Verification items for this drawing (mm, ordinates from the low corner). Give positions to 0.01 mm unless a question says otherwise; leave off trailing zeros. Loops run counter-clockwise (first coordinate to the right, second up) from the corner with the lowest first, then second, coordinate; pieces in that order, holes last. Notation, with made-up numbers: (44, -32) -> (94, -32) arc R16 cw to (94, -2) -> close; hole circle Ø2 at (83.5, 33). An arc over 180 degrees is marked (long way). Answer as a JSON object with one key per item and string values.
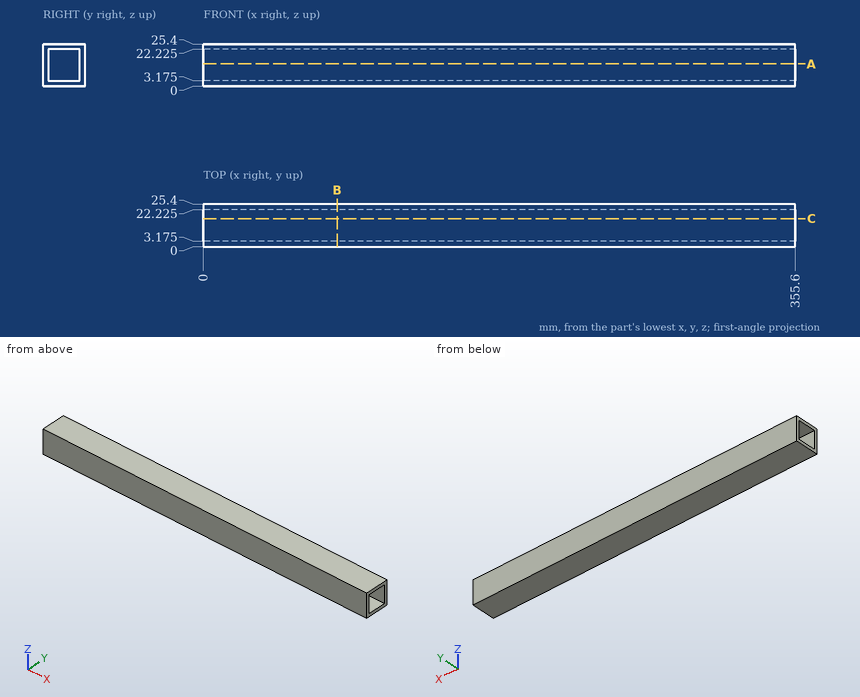
1) Depth check by flat-ended pin: P1, Ø10, axis at y = 18.5, z = 5, coming from the -X side. Enter the tip coordinate at first touch or a pass-through.
Geometry check:
{"P1": "stops at x = 0"}
2) Section check B-B on x = 80.5. Record the cut outline in (y, z) (3 decimals).
Geometry check:
{"outline": "(0, 0) -> (25.4, 0) -> (25.4, 25.4) -> (0, 25.4) -> close; hole (3.175, 3.175) -> (22.225, 3.175) -> (22.225, 22.225) -> (3.175, 22.225) -> close"}
3) Material ranges on line 1 along Y through (x, z) = (73, 21.75) (3 decimals), recorded low to high. Write a range as from..to.
Geometry check:
{"line 1": "y = 0..3.175, 22.225..25.4"}
4) Section check A-A on z = 13.5. Record the cut outline in (x, y) (3 decimals).
Geometry check:
{"outline": "(0, 0) -> (355.6, 0) -> (355.6, 3.175) -> (0, 3.175) -> close; (0, 22.225) -> (355.6, 22.225) -> (355.6, 25.4) -> (0, 25.4) -> close"}
